```python
from build123d import *

# Parameters (mm, degrees)
F0_R     = 15.875
F1_DEPTH = 22.225
F3_R     = 0.889
F5_DEPTH = 23.749
F9_W     = 21.712904
F9_H     = 4.7625
F7_DEPTH = 22.225
F6_W     = 16.982072
F6_H     = 4.7625
F8_DEPTH = 22.225


with BuildPart() as f1:
    # F0 (on Top) → F1 (new body)
    with BuildSketch(Plane.XY):
        Circle(F0_R)
    extrude(amount=F1_DEPTH)

    # F3 (on face) → F5 (join)
    with BuildSketch(Plane(origin=(0, 0, 0), x_dir=(1, 0, 0), z_dir=(0, 0, -1))):
        with Locations((0, 13.652203)):
            Circle(F3_R)
        with Locations((-13.659894, -0.015021)):
            Circle(F3_R)
        with Locations((0.062219, -13.682245)):
            Circle(F3_R)
        with Locations((13.674476, -0.124876)):
            Circle(F3_R)
    extrude(amount=-F5_DEPTH)

    # F9 (on face) → F7 (cut)
    with BuildSketch(Plane.XY.offset(22.225)):
        with Locations((0.014928, 0.097281)):
            Rectangle(F9_W, F9_H)
    extrude(amount=-F7_DEPTH, mode=Mode.SUBTRACT)

    # F6 (on face) → F8 (cut)
    with BuildSketch(Plane.XY.offset(22.225)):
        with Locations((-0.042667, 6.022512)):
            Rectangle(F6_W, F6_H)
        with Locations((-0.042667, -6.022512)):
            Rectangle(F6_W, F6_H)
    extrude(amount=-F8_DEPTH, mode=Mode.SUBTRACT)


solid = f1.part
```
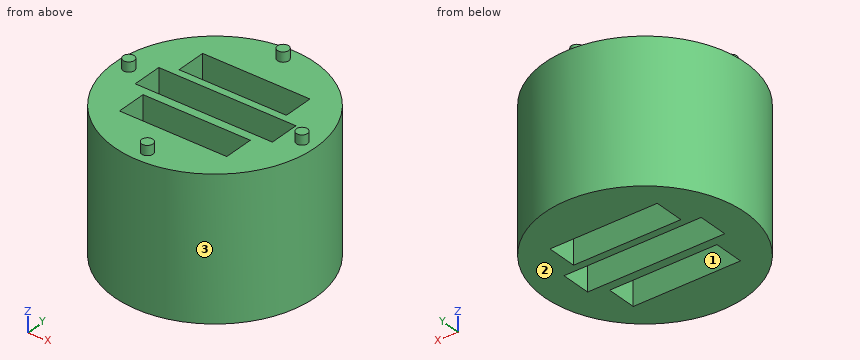
The listing builds one solid part. Answer for the finished solid, in the listing's coordinates (mm). Face numbers are marked on the shaded views. Give positions to 0.01 mm unless a question says otherwise; leave off trailing zeros. Order: outer loops, then holes, each group sorted by start corner. A loop starts at its lowest first (then second) coordinate and runs counter-clockwise, first axis right, second up. Notation, with made-up numbers: M 5,6 L 48,6 A12 cw 48,26 Z; hole C 48,40 d9. An arc over 180 degrees is marked long. Put each result on its own line as item: value. Start each with the question number.
Item 1: For a pull along X with two mould halves and no side action, classify the marked faces 1, 2 and 3 as +X half, -X half, draft (parallel to the pull), parting line (faces both ways), or undercut.
Item 2: The part is cut by section B-B, the plane x = 0. Determine the outline of the cut face in (y, z) (3 decimals).
Item 3: The part is cut by section C-C, the plane y = 3. Determine the outline of the cut face in (x, z) (3 decimals).
Item 4: The part is cut by section A-A, the plane z = 13.5. Determine the outline of the cut face in (x, y) (3 decimals).
Item 5: The part is cut by section D-D, the plane x = 6. Determine the outline of the cut face in (y, z) (3 decimals).
Item 6: Flat-ended cylindrical pins translate along their axes: P1, Ø8, axis at x = -8, z = 18, coming from the -Y side; P2, Ø2.5, axis at y = 7, z = 7.5, coming from the -X side; P3, Ø2.5, axis at y = -6, z = 12, coming from the +X side. Find the tip coordinate at first contact, or state that the pin passes through.
Item 7: Find the intervals of material crossed by line 1 along Y through (x, z) = (0, 19) (3 decimals); line 2 along Y through (x, z) = (-8, 16.75); line 3 along Z through (x, y) = (-13, -2) (3 decimals), in increasing order.
Answer key:
1. face 1: undercut
1. face 2: draft
1. face 3: parting line
2. outline: M -15.875,0 L -8.404,0 L -8.404,22.225 L -12.763,22.225 L -12.763,23.749 L -14.541,23.749 L -14.541,22.225 L -15.875,22.225 Z; M -3.641,0 L -2.284,0 L -2.284,22.225 L -3.641,22.225 Z; M 2.479,0 L 3.641,0 L 3.641,22.225 L 2.479,22.225 Z; M 8.404,0 L 15.875,0 L 15.875,22.225 L 14.569,22.225 L 14.569,23.749 L 12.795,23.749 L 12.795,22.225 L 8.404,22.225 Z
3. outline: M -15.589,0 L 15.589,0 L 15.589,22.225 L -15.589,22.225 Z
4. outline: C 0,0 d31.75; hole M -10.842,-2.284 L 10.871,-2.284 L 10.871,2.479 L -10.842,2.479 Z; hole M -8.534,-8.404 L 8.448,-8.404 L 8.448,-3.641 L -8.534,-3.641 Z; hole M -8.534,3.641 L 8.448,3.641 L 8.448,8.404 L -8.534,8.404 Z
5. outline: M -14.697,0 L -8.404,0 L -8.404,22.225 L -14.697,22.225 Z; M -3.641,0 L -2.284,0 L -2.284,22.225 L -3.641,22.225 Z; M 2.479,0 L 3.641,0 L 3.641,22.225 L 2.479,22.225 Z; M 8.404,0 L 14.697,0 L 14.697,22.225 L 8.404,22.225 Z
6. P1: stops at y = -15.36
6. P2: stops at x = -14.8
6. P3: stops at x = 15.15
7. line 1: y = -15.875 to -8.404, -3.641 to -2.284, 2.479 to 3.641, 8.404 to 15.875
7. line 2: y = -13.71 to -8.4, -3.64 to -2.28, 2.48 to 3.64, 8.4 to 13.71
7. line 3: z = 0 to 22.225
